```python
from build123d import *

# Parameters (mm, degrees)
SKETCH2_R                    = 55
SKETCH2_R_2                  = 50
BOSS_EXTRUDE1_DEPTH          = 20
SKETCH3_R                    = 55
BOSS_EXTRUDE2_DEPTH          = 5
TAP_DRILL_FOR_M14X2_0_TAP1_D = 14
CIRPATTERN1_COUNT            = 3


with BuildPart() as part:
    # Sketch2 → Boss-Extrude1 (new body)
    with BuildSketch(Plane(origin=(0, 0, 0), x_dir=(1, 0, 0), z_dir=(0, 1, 0))):
        Circle(SKETCH2_R)
        Circle(SKETCH2_R_2, mode=Mode.SUBTRACT)
    extrude(amount=-BOSS_EXTRUDE1_DEPTH)

    # Sketch3 → Boss-Extrude2 (add)
    with BuildSketch(Plane(origin=(0, 0, 0), x_dir=(1, 0, 0), z_dir=(0, 1, 0))):
        Circle(SKETCH3_R)
    extrude(amount=-BOSS_EXTRUDE2_DEPTH)

    # Tap Drill for M14x2.0 Tap1 (through all)
    with Locations(Plane(origin=(0, 0, 0), x_dir=(1, 0, 0), z_dir=(0, 1, 0))):
        with Locations((42, 0)):
            tap_drill_for_m14x2_0_tap1 = Hole(TAP_DRILL_FOR_M14X2_0_TAP1_D / 2)

    # CirPattern1: Tap Drill for M14x2.0 Tap1 ×3 about axis
    cirpattern1_axis = Axis((0, 0, 0), (0, 1, 0))
    for i in range(1, CIRPATTERN1_COUNT):
        add(tap_drill_for_m14x2_0_tap1.rotate(cirpattern1_axis, i * 360 / CIRPATTERN1_COUNT), mode=Mode.SUBTRACT)


solid = part.part
```
Check sheet for the modelled part. Datum: model origin and axes. Units: mm. A direction names the side the tool comes from. Coordinates: 2 decimals unless noted, no trailing zeros. Write each loop counter-clockwise with the first axis right and the second up, starting at its lowest first coordinate (ties: lowest second). Pieces come first, ordered by that corner, then holes. Notation, with made-up numbers: (42, -23) -> (90, -23) arc R26 ccw to (90, -7) -> close; hole circle Ø10 at (48.25, -0.5). An arc over 180 degrees is marked (long way). Use a Markdown table: item, result.
1. Scan lines: line 1 along X through (y, z) = (-10, 0); line 2 along Z through (x, y) = (-21, -3.05); line 3 along Z through (x, y) = (-15, -2.75). Record each from-to range of solid material in increasing order.
Reported:
| item | result |
|---|---|
| line 1 | x = -55 to -50, 50 to 55 |
| line 2 | z = -50.83 to -43.37, -29.37 to 29.37, 43.37 to 50.83 |
| line 3 | z = -52.92 to -39.98, -32.77 to 32.77, 39.98 to 52.92 |
2. Sectioned sample at D-D (x = -21). Enter the section's corners in (y, z), plus the area to 3 significant figures.
Reported:
| item | result |
|---|---|
| outline | (-20, -50.83) -> (0, -50.83) -> (0, -43.37) -> (-5, -43.37) -> (-5, -45.38) -> (-20, -45.38) -> close; (-20, 45.38) -> (-5, 45.38) -> (-5, 43.37) -> (0, 43.37) -> (0, 50.83) -> (-20, 50.83) -> close; (-5, -29.37) -> (0, -29.37) -> (0, 29.37) -> (-5, 29.37) -> close |
| area | 532 mm2 |
3. Go/stop test with flat-tipped pins: pin 1 Ø3 at (x, y) = (-11, -5.5) entering from -Z; pin 2 Ø4 at (y, z) = (-7, 5.5) entering from -X; pin 3 Ø12 at (y, z) = (-4.5, -41.5) entering from -X. Record where each tip stops, or that it passes through.
Reported:
| item | result |
|---|---|
| pin 1 | stops at z = -54.17 |
| pin 2 | stops at x = -54.89 |
| pin 3 | stops at x = -42.01 |
4. Sectioned sample at B-B (x = 0). Enter the section's corners in (y, z), plus the area to 3 significant figures.
Reported:
| item | result |
|---|---|
| outline | (-20, -55) -> (0, -55) -> (0, 55) -> (-20, 55) -> (-20, 50) -> (-5, 50) -> (-5, -50) -> (-20, -50) -> close |
| area | 700 mm2 |
5. Sectioned sample at C-C (y = -14.5). Enter the section's corners in (x, z).
Reported:
| item | result |
|---|---|
| outline | circle Ø110 at (0, 0); hole circle Ø100 at (0, 0) |
6. Tool access check on faces 4 (the flat face through (-1, 0, -1)), 5 (the cylindrical face through (47.69, -12.4, -15.02)). Record the directions out of +Z, -Z, +X, -X, +Y, -Y that give a thin tool (end or side, any length) a straight path to the whole face; none if there is none.
Reported:
| item | result |
|---|---|
| face 4 | +Z, -Z, +X, -X, +Y |
| face 5 | -Y |
7. Release check for a two-part mould opening along Z. For faces 1 (the flat face through (12, -20, 49)), 2 (the cylindrical face through (-11.923, -9.86, 53.692)), 3 (the cylindrical face through (-15.445, -2.535, 40.632)) record: pulls with the +Z half, pulls with the -Z half, needs draft (parallel to the pull), parting line crosses it, or undercut.
Reported:
| item | result |
|---|---|
| face 1 | needs draft |
| face 2 | parting line crosses it |
| face 3 | undercut |
8. Sectioned sample at A-A (z = 0). Enter the section's corners in (x, y), plus the area to 3 significant figures.
Reported:
| item | result |
|---|---|
| outline | (-55, -20) -> (-50, -20) -> (-50, -5) -> (35, -5) -> (35, 0) -> (-55, 0) -> close; (49, -5) -> (50, -5) -> (50, -20) -> (55, -20) -> (55, 0) -> (49, 0) -> close |
| area | 630 mm2 |
